Input: part model. Units: mm. Frame: model coordinates. Face numbers are marked on the shaded views. Give positions to 0.01 mm unless a question says otherwise; leave off trailing zeros. Order: outer loops, then holes, each group sorted by start corner. A loop starts at its lowest first (then second) coordinate and runs counter-clockwise, first axis right, second up. Notation, with made-up numbers: M 64,3.25 L 78,3.25 A12 cw 78,23.25 Z; hole C -9.75,62 d7. An arc over 180 degrees is marked long. Use a Markdown table: item, result.
from build123d import *

# Parameters (mm, degrees)
F0_W     = 71
F0_H     = 130.5
F1_DEPTH = 10
F2_SIZE  = 3.5
F3_R     = 2
F4_T     = 2
F5_R     = 1.6
F6_DEPTH = 5
F7_SIZE  = 1.6
F8_R     = 5


# Not quite as in the source:
# - a shell that OpenCascade refuses in one call is made with other operations: the cavity is built on its own and cut out


with BuildPart() as f1:
    # F0 (on Top) → F1 (new body)
    with BuildSketch(Plane.XY):
        Rectangle(F0_W, F0_H)
    extrude(amount=F1_DEPTH)

    # F2
    f2_edges = [f1.edges().sort_by_distance(p)[0] for p in [
        (-35.5, -65.25, 5),
        (35.5, -65.25, 5),
        (-35.5, 65.25, 5),
        (35.5, 65.25, 5),
    ]]
    chamfer(f2_edges, length=F2_SIZE)

    # F3
    f3_edges = [f1.edges().sort_by_distance(p)[0] for p in [
        (-32, 65.25, 5),
        (-35.5, 61.75, 5),
        (32, 65.25, 5),
        (35.5, 61.75, 5),
        (32, -65.25, 5),
        (35.5, -61.75, 5),
        (-35.5, -61.75, 5),
        (-32, -65.25, 5),
    ]]
    fillet(f3_edges, radius=F3_R)

    # F4: shell of thickness 2, made by hand


with BuildPart() as f4_core1:
    # F4_t2: copy of F1
    add(f1.part)

    # the walls: a layer under each face that stays
    f4_faces = [f4_core1.faces().sort_by_distance(p)[0] for p in [
        (0, -65.25, 5),
        (0, 0, 0),
        (-33.75, -63.5, 5),
        (33.75, -63.5, 5),
        (-35.5, 0, 5),
        (35.5, 0, 5),
        (-33.75, 63.5, 5),
        (33.75, 63.5, 5),
        (0, 65.25, 5),
    ]]
    thicken(f4_faces, amount=-F4_T, mode=Mode.SUBTRACT)


with BuildPart() as f1_1:
    add(f1.part)

    # what is left inside the walls is the cavity
    f4_cavity = [f4_core1.part.solids().sort_by_distance(p)[0] for p in [
        (0, -21.083333, 2.02),
    ]]
    add(f4_cavity, mode=Mode.SUBTRACT)

    # F5 (on face) → F6 (join)
    with BuildSketch(Plane.XY.offset(2)):
        with Locations((-27, -3.25)):
            Circle(F5_R)
        with Locations((-15.5, -11.25)):
            Circle(F5_R)
        with Locations((-3.5, -18.25)):
            Circle(F5_R)
        with Locations((6.5, -24.25)):
            Circle(F5_R)
        with Locations((16.5, -15.25)):
            Circle(F5_R)
        with Locations((28, -8.25)):
            Circle(F5_R)
    extrude(amount=F6_DEPTH)

    # F7
    f7_edges = [f1_1.edges().sort_by_distance(p)[0] for p in [
        (-28.6, -3.25, 7),
        (-17.1, -11.25, 7),
        (-5.1, -18.25, 7),
        (4.9, -24.25, 7),
        (14.9, -15.25, 7),
        (26.4, -8.25, 7),
    ]]
    chamfer(f7_edges, length=F7_SIZE)

    # F8
    f8_edges = [f1_1.edges().sort_by_distance(p)[0] for p in [
        (-28.6, -3.25, 5.4),
        (-17.1, -11.25, 5.4),
        (-5.1, -18.25, 5.4),
        (4.9, -24.25, 5.4),
        (14.9, -15.25, 5.4),
        (26.4, -8.25, 5.4),
    ]]
    fillet(f8_edges, radius=F8_R)


solid = f1_1.part
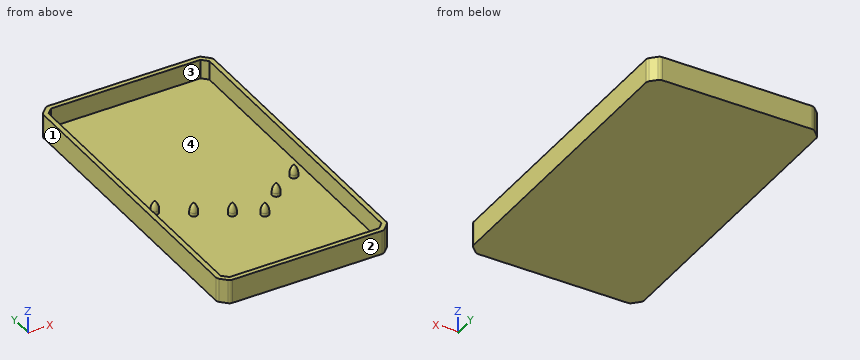
1) Cut plane A-A on x = 10. Return loops of the section in (y, z), and give its area (3 significant figures).
Response values:
| item | result |
|---|---|
| outline | M -65.25,0 L 65.25,0 L 65.25,10 L 63.25,10 L 63.25,2 L -63.25,2 L -63.25,10 L -65.25,10 Z |
| area | 293 mm² |
2) Material intervals for line 1 (Y direction, x = 22, z = 7.5); line 2 (X direction, y = 25, z = 8); line 3 (Y direction, x = 27.5, z = 4), sorted ascending. Write a range as from..to.
Response values:
| item | result |
|---|---|
| line 1 | y = -65.25..-63.25, 63.25..65.25 |
| line 2 | x = -35.5..-33.5, 33.5..35.5 |
| line 3 | y = -65.25..-63.25, -9.72..-6.78, 63.25..65.25 |
3) Mould query, pull axis X, two halves, no side actions, for the marked faces 1, 2, 3 and 4. Classes: released by +X, released by -X, zero draft, split by the parting line, or undercut.
Response values:
| item | result |
|---|---|
| face 1 | released by -X |
| face 2 | zero draft |
| face 3 | undercut |
| face 4 | undercut |
4) Cut plane C-C on z = 5. State how many separate pieces and enclosed holes the cut face has, and give its area (3 significant figures).
Response values:
| item | result |
|---|---|
| separate pieces | 7 |
| enclosed holes | 1 |
| area | 808 mm² |
5) First-contact query: pin 1 Ø12 at (x, y) = (-6.5, 35.5) entering from +Z; pin 2 Ø5 at (x, y) = (-7, 4) entering from -Z. Flat tips, straight axial feed; report the tip coordinate or a pass-through.
Response values:
| item | result |
|---|---|
| pin 1 | stops at z = 2 |
| pin 2 | stops at z = 0 |
6) Cut plane B-B on y = 6. Return loops of the section in (x, z).
Response values:
| item | result |
|---|---|
| outline | M -35.5,0 L 35.5,0 L 35.5,10 L 33.5,10 L 33.5,2 L -33.5,2 L -33.5,10 L -35.5,10 Z |
